Here's how the part is built. I have some questions about the finished solid (model axes, mm). A direction names the side the tool comes from. Give positions to 0.01 mm unless a question says otherwise; leave off trailing zeros. Loops run counter-clockwise (first coordinate to the right, second up) from the corner with the lowest first, then second, coordinate; pieces in that order, holes last. Notation, with made-up numbers: (16, -20) -> (66, -20) arc R21 ccw to (66, 13) -> close; hole circle Ø5 at (35.25, 8.5). An arc over 180 degrees is marked (long way). Answer in a Markdown table with one row per item. Add a question column.
Item 1: For P1, Ø4.5, axis at x = 2.5, y = 2, coming from the -Z side; P2, Ø13.5, axis at x = 6.5, z = -40, coming from the -Y side; P3, Ø5, axis at x = 10, z = -29.5, coming from the +Y side; P4, Ø3, axis at x = -9, z = -38.5, coming from the +Y side, each with a flat end and sliding along its axis, tell me the tip position at first contact or that it passes through.
Item 2: Which directions (+Z, -Z, +X, -X, +Y, -Y) give clear straight access to the entire face, cutting with the end or side of a thin tool? Please do faces 4 (the face through (-13.45, 7.99, 0.96)), 5 (the face through (-0.329, 8.72, 8.116)), 6 (the face through (0, 2, 0)).
Item 3: If we section it at B-B (y = 2): Write out the boundary of the cut face in (x, z).
Item 4: We'd pull the mould along Y, two halves only. Please class faces 1 (the face through (-0.329, 7.395, -23.351)), 2 (the face through (-14.75, 5.42, 2.69)), 3 (the face through (-0.329, 3.398, 4.223)): released by +Y, released by -Y, zero draft, split by the parting line, or undercut.
Item 5: If we section it at C-C (z = -16): Write out the boundary of the cut face in (x, y), then the cut area to 3 significant figures.
Item 6: If we section it at A-A (x = 10): Write out the boundary of the cut face in (y, z).
Item 7: If I drill on line 1 (X direction, y = 2, z = -15); line 2 (X direction, y = 5.5, z = -10); line 3 (X direction, y = 4.75, z = -39.5), over which ranges is the centre line in solid material (lowest first)?
Item 8: If we section it at D-D (z = -40): Give the number of separate pieces and of enclosed holes in the cut face, then the cut area to 3 significant figures.
```python
from build123d import *

# Parameters (mm, degrees)
BOSS_EXTRU_1_DEPTH                            = 23.5
BOSS_EXTRU_1_DEPTH_BACK                       = 23.5
ESQUISSE2_W                                   = 45.2
ESQUISSE2_H                                   = 53.75
ENL_V_MAT_EXTRU_1_DEPTH                       = 4.05
ENL_V_MAT_EXTRU_2_REACH                       = 60.542
ESQUISSE3_R                                   = 1.6
TROU_POUR_TARAUDAGE_POUR_TROU_TARAUD_M3_D     = 2.5
TROU_POUR_TARAUDAGE_POUR_TROU_TARAUD_M3_DEPTH = 5
TROU_POUR_TARAUDAGE_POUR_TROU_TARAUD_M3_TIP   = 0.751075774


with BuildPart() as part:
    # Esquisse1 → Boss.-Extru.1 (new, two sides: drawn at the far end of the back side and taken through both)
    with BuildSketch(Plane(origin=(0, 0, 0), x_dir=(0, 0, -1), z_dir=(1, 0, 0)).offset(-BOSS_EXTRU_1_DEPTH_BACK)):
        Polygon((53.75, 4.2), (-7.910357513, 10.680764723), (-8.328471366, 6.702677141), (0, 0), (53.75, 0), align=None)
    extrude(amount=BOSS_EXTRU_1_DEPTH + BOSS_EXTRU_1_DEPTH_BACK)

    # Esquisse2 → Enlèv. mat.-Extru.1 (cut)
    with BuildSketch(Plane.XZ):
        with Locations((0, -26.875)):
            Rectangle(ESQUISSE2_W, ESQUISSE2_H)
    extrude(amount=-ENL_V_MAT_EXTRU_1_DEPTH, mode=Mode.SUBTRACT)

    # Enlèv. mat.-Extru.2: up to this plane
    enl_v_mat_extru_2_end = Plane(origin=(0, 4.05, 0), z_dir=(0, -1, 0))
    # Esquisse3 → Enlèv. mat.-Extru.2 (cut, up to the surface)
    with BuildSketch(Plane(origin=(0, 9.741736652, -1.023897781), x_dir=(1, 0, 0), z_dir=(0, 0.9945218953682741, -0.10452846326764641)), mode=Mode.PRIVATE) as enl_v_mat_extru_2_sk1:
        with Locations(Location((-15.5, 39.929033745, 0), (0, 0, 270))):
            Circle(ESQUISSE3_R)
    enl_v_mat_extru_2_tool1 = split(extrude(enl_v_mat_extru_2_sk1.sketch, amount=-ENL_V_MAT_EXTRU_2_REACH, mode=Mode.PRIVATE), bisect_by=enl_v_mat_extru_2_end, keep=Keep.BOTH, mode=Mode.PRIVATE)
    add(enl_v_mat_extru_2_tool1.solids().sort_by_distance((-15.5, 5.568016, -40.734196))[0], mode=Mode.SUBTRACT)
    # Esquisse3 → Enlèv. mat.-Extru.2 (cut, up to the surface)
    with BuildSketch(Plane(origin=(0, 9.741736652, -1.023897781), x_dir=(1, 0, 0), z_dir=(0, 0.9945218953682741, -0.10452846326764641)), mode=Mode.PRIVATE) as enl_v_mat_extru_2_sk2:
        with Locations(Location((15.5, 39.929033745, 0), (0, 0, 270))):
            Circle(ESQUISSE3_R)
    enl_v_mat_extru_2_tool2 = split(extrude(enl_v_mat_extru_2_sk2.sketch, amount=-ENL_V_MAT_EXTRU_2_REACH, mode=Mode.PRIVATE), bisect_by=enl_v_mat_extru_2_end, keep=Keep.BOTH, mode=Mode.PRIVATE)
    add(enl_v_mat_extru_2_tool2.solids().sort_by_distance((15.5, 5.568016, -40.734196))[0], mode=Mode.SUBTRACT)
    # Esquisse3 → Enlèv. mat.-Extru.2 (cut, up to the surface)
    with BuildSketch(Plane(origin=(0, 9.741736652, -1.023897781), x_dir=(1, 0, 0), z_dir=(0, 0.9945218953682741, -0.10452846326764641)), mode=Mode.PRIVATE) as enl_v_mat_extru_2_sk3:
        with Locations(Location((15.5, 7.929033745, 0), (0, 0, 270))):
            Circle(ESQUISSE3_R)
    enl_v_mat_extru_2_tool3 = split(extrude(enl_v_mat_extru_2_sk3.sketch, amount=-ENL_V_MAT_EXTRU_2_REACH, mode=Mode.PRIVATE), bisect_by=enl_v_mat_extru_2_end, keep=Keep.BOTH, mode=Mode.PRIVATE)
    add(enl_v_mat_extru_2_tool3.solids().sort_by_distance((15.5, 8.912927, -8.909495))[0], mode=Mode.SUBTRACT)
    # Esquisse3 → Enlèv. mat.-Extru.2 (cut, up to the surface)
    with BuildSketch(Plane(origin=(0, 9.741736652, -1.023897781), x_dir=(1, 0, 0), z_dir=(0, 0.9945218953682741, -0.10452846326764641)), mode=Mode.PRIVATE) as enl_v_mat_extru_2_sk4:
        with Locations(Location((-15.5, 7.929033745, 0), (0, 0, 270))):
            Circle(ESQUISSE3_R)
    enl_v_mat_extru_2_tool4 = split(extrude(enl_v_mat_extru_2_sk4.sketch, amount=-ENL_V_MAT_EXTRU_2_REACH, mode=Mode.PRIVATE), bisect_by=enl_v_mat_extru_2_end, keep=Keep.BOTH, mode=Mode.PRIVATE)
    add(enl_v_mat_extru_2_tool4.solids().sort_by_distance((-15.5, 8.912927, -8.909495))[0], mode=Mode.SUBTRACT)

    # Trou pour taraudage pour trou taraudé M31
    with Locations(Plane(origin=(0, 0, 0), x_dir=(-1, 0, 0), z_dir=(0, -0.779044883952261, 0.6269681561194383))):
        with Locations((13.5, -5.548250916), (-13.5, -5.548250916)):
            Hole(TROU_POUR_TARAUDAGE_POUR_TROU_TARAUD_M3_D / 2, depth=TROU_POUR_TARAUDAGE_POUR_TROU_TARAUD_M3_DEPTH)
            with Locations((0, 0, -(TROU_POUR_TARAUDAGE_POUR_TROU_TARAUD_M3_DEPTH + TROU_POUR_TARAUDAGE_POUR_TROU_TARAUD_M3_TIP / 2))):  # 118° drill point
                Cone(0, TROU_POUR_TARAUDAGE_POUR_TROU_TARAUD_M3_D / 2, TROU_POUR_TARAUDAGE_POUR_TROU_TARAUD_M3_TIP, mode=Mode.SUBTRACT)


solid = part.part
```
Recorded:
| question | item | result |
|---|---|---|
| 1 | P1 | stops at z = -53.75 |
| 1 | P2 | stops at y = 4.05 |
| 1 | P3 | stops at y = 7.01 |
| 1 | P4 | stops at y = 5.96 |
| 2 | face 4 | none |
| 2 | face 5 | +Z, +X, -X, +Y |
| 2 | face 6 | -Z, -Y |
| 3 | outline | (-23.5, -53.75) -> (-22.6, -53.75) -> (-22.6, 0) -> (22.6, 0) -> (22.6, -53.75) -> (23.5, -53.75) -> (23.5, 2.49) -> (-23.5, 2.49) -> close |
| 4 | face 1 | released by +Y |
| 4 | face 2 | undercut |
| 4 | face 3 | released by -Y |
| 5 | outline | (-23.5, 0) -> (-22.6, 0) -> (-22.6, 4.05) -> (22.6, 4.05) -> (22.6, 0) -> (23.5, 0) -> (23.5, 8.17) -> (-23.5, 8.17) -> close |
| 5 | area | 201 mm^2 |
| 6 | outline | (0, 0) -> (4.05, 0) -> (4.05, -53.75) -> (4.2, -53.75) -> (10.68, 7.91) -> (6.7, 8.33) -> close |
| 7 | line 1 | x = -23.5 to -22.6, 22.6 to 23.5 |
| 7 | line 2 | x = -23.5 to -16.19, -14.81 to 14.81, 16.19 to 23.5 |
| 7 | line 3 | x = -23.5 to -16.62, -14.38 to 14.38, 16.62 to 23.5 |
| 8 | separate pieces | 3 |
| 8 | enclosed holes | 0 |
| 8 | area | 73.0 mm^2 |
